For this review, take the finished solid that the model builds, in its own axes (mm). A direction names the side the tool comes from. Coordinates: 2 decimals unless noted, no trailing zeros. Write each loop counter-clockwise with the first axis right and the second up, starting at its lowest first coordinate (ties: lowest second). Pieces come first, ordered by that corner, then holes.
```python
from build123d import *

# Parameters (mm, degrees)
F1_DEPTH = 101.6
F2_DEPTH = 105.41
F3_R     = 3.80999
F4_R     = 3.80999
F5_DEPTH = 109.22
F6_R     = 3.80999


# Not quite as in the source:
# - a fillet or chamfer is up to 0.001 mm smaller than in the source, because OpenCascade refuses the exact size


with BuildPart() as f1:
    # F0 (on Right) → F1 (new body, symmetric)
    with BuildSketch(Plane.YZ):
        Polygon((-28.9227480759, 13.4151088954), (-34.29, 1.905), (-19.7165844463, 1.905), (3.9163465702, 52.5859841168), (30.004847431, 1.905), (34.29, 1.905), (3.7473661652, 61.2388325007), (-23.0888934554, 3.6882880238), (-28.1533413693, 6.0498788705), (-25.4697154073, 11.8049333181), align=None)
    extrude(amount=F1_DEPTH, both=True)

    # F0 (on Right) → F2 (join, symmetric)
    with BuildSketch(Plane.YZ):
        Polygon((-38.1, 1.905), (-38.1, -1.905), (38.1, -1.905), (38.1, 1.905), (34.29, 1.905), (30.004847431, 1.905), (-19.7165844463, 1.905), (-34.29, 1.905), align=None)
    extrude(amount=F2_DEPTH, both=True)

    # F3 (radius 3.81 in the source; OpenCascade refuses exactly that, so slightly less here)
    f3_edges = [f1.edges().sort_by_distance(p)[0] for p in [
        (-105.41, 0, 1.905),
        (0, -38.1, 1.905),
        (0, 38.1, 1.905),
        (105.41, 0, 1.905),
    ]]
    fillet(f3_edges, radius=F3_R)

    # F4 (radius 3.81 in the source; OpenCascade refuses exactly that, so slightly less here)
    f4_edges = [f1.edges().sort_by_distance(p)[0] for p in [
        (0, -28.922748, 13.415109),
    ]]
    fillet(f4_edges, radius=F4_R)

    # F0 (on Right) → F5 (join, symmetric)
    with BuildSketch(Plane.YZ):
        Polygon((38.1, -1.905), (-38.1, -1.905), (-41.91, -1.905), (-41.91, -5.715), (41.91, -5.715), (41.91, -1.905), align=None)
    extrude(amount=F5_DEPTH, both=True)

    # F6 (radius 3.81 in the source; OpenCascade refuses exactly that, so slightly less here)
    f6_edges = [f1.edges().sort_by_distance(p)[0] for p in [
        (-109.22, 0, -1.905),
        (0, 41.91, -1.905),
        (109.22, 0, -1.905),
        (0, -41.91, -1.905),
    ]]
    fillet(f6_edges, radius=F6_R)


solid = f1.part
```
Q1. Clearance check with flat-ended pins moving along their axes: pin 1 Ø2 at (x, z) = (-52, 15.5) entering from +Y; pin 2 Ø2 at (x, y) = (1.5, 25) entering from +Z; pin 3 Ø5 at (x, z) = (-57, 38) entering from +Y; pin 4 Ø10 at (y, z) = (-12.5, 40) entering from +X. State where each tip first meets the part, or that it passes through.
Ans:
pin 1: stops at y = 27.81
pin 2: stops at z = 21.89
pin 3: stops at y = 17
pin 4: passes through
Q2. Draft analysis for pull direction Z (two halves, no side actions). For faces 4 (the flat face through (1, 8, 1.905)), 5 (the flat face through (101.6, -8, 30)), 6 (the flat face through (1.42, -9.48, 32.87)), state which applies: +Z half, -Z half, draft (parallel to the pull), parting line (faces both ways), or undercut.
Ans:
face 4: undercut
face 5: draft
face 6: +Z half
Q3. Add section C-C (z = 37.5). State the section outline as (x, y) points.
Ans:
outline: (-101.6, -7.32) - (101.6, -7.32) - (101.6, -3.12) - (-101.6, -3.12) - close; (-101.6, 11.68) - (101.6, 11.68) - (101.6, 15.97) - (-101.6, 15.97) - close
Q4. Tool access review of faces 1 (the flat face through (-101.6, -8, 30)), 2 (the flat face through (1.42, 16.78, 27.6)), 3 (the cylindrical face through (-1.53, 40.76, -2.99)): name each direction out of +Z, -Z, +X, -X, +Y, -Y from which nothing blocks a thin tool from reaching the whole face with its end or side.
Ans:
face 1: +Z, -X, +Y, -Y
face 2: +X, -X
face 3: +Z, +X, -X, +Y
Q5. For probe 1 along Z at (x, y) = (-56.5, 38.5) (3 decimals); probe 2 along Y at (x, z) = (39, 25); probe 3 along Y at (x, z) = (34, 40), list the stretches that pass through material, from the lowest coordinate up.
Ans:
probe 1: z = -5.715 to -1.926
probe 2: y = -13.15 to -8.95, 18.12 to 22.4
probe 3: y = -6.16 to -1.95, 10.4 to 14.68
